from build123d import *

# Parameters (mm, degrees)
BOSS_EXTRUDE1_DEPTH     = 3
SKETCH2_R               = 0.875
CUT_EXTRUDE1_DEPTH      = 51
CUT_EXTRUDE1_DEPTH_BACK = 3
FILLET2_R               = 1.5
CHAMFER1_SIZE           = 1.5


with BuildPart() as part:
    # Sketch1 → Boss-Extrude1 (new body)
    with BuildSketch(Plane(origin=(0, 0, 0), x_dir=(1, 0, 0), z_dir=(0, 1, 0))):
        Polygon((-25, -21), (-20, -21), (-20, 11), (20, 11), (20, -21), (25, -21), (25, 14), (-25, 14), align=None)
    extrude(amount=BOSS_EXTRUDE1_DEPTH)

    # Sketch2 → Cut-Extrude1 (cut, two sides)
    with BuildSketch(Plane.ZY.offset(-25)) as cut_extrude1_sk:
        with Locations((18, 1.5)):
            Circle(SKETCH2_R)
        with Locations((13, 1.5)):
            Circle(SKETCH2_R)
        with Locations((8, 1.5)):
            Circle(SKETCH2_R)
        with Locations((3, 1.5)):
            Circle(SKETCH2_R)
        with Locations((-2, 1.5)):
            Circle(SKETCH2_R)
        with Locations((-7, 1.5)):
            Circle(SKETCH2_R)
    extrude(amount=CUT_EXTRUDE1_DEPTH, mode=Mode.SUBTRACT)
    extrude(cut_extrude1_sk.sketch, amount=-CUT_EXTRUDE1_DEPTH_BACK, mode=Mode.SUBTRACT)

    # Fillet2
    fillet2_edges = [part.edges().sort_by_distance(p)[0] for p in [
        (25, 1.5, 21),
        (-25, 1.5, 21),
        (-25, 1.5, -14),
        (25, 1.5, -14),
    ]]
    fillet(fillet2_edges, radius=FILLET2_R)

    # Chamfer1
    chamfer1_edges = [part.edges().sort_by_distance(p)[0] for p in [
        (20, 1.5, -11),
        (-20, 1.5, -11),
    ]]
    chamfer(chamfer1_edges, length=CHAMFER1_SIZE)


solid = part.part
Verification items for the finished model (mm, model axes). A direction names the side the tool comes from. Give positions to 0.01 mm unless a question says otherwise; leave off trailing zeros. Loops run counter-clockwise (first coordinate to the right, second up) from the corner with the lowest first, then second, coordinate; pieces in that order, holes last.
1) Thickness scan on line 1 along X through (y, z) = (0.7, 5); line 2 along Y through (x, z) = (22, 3) (3 decimals); line 3 along Z through (x, y) = (12, 1.8). Record the ranges inside material, lowest first.
2) Sectioned sample at B-B, the plane z = 8. Enter the section's corners in (x, y) (3 decimals).
3) Sectioned sample at C-C, the plane y = 1.5. Count the separate pieces of the cut face and the enclosed holes in it, then the cut area to 3 significant figures.
4) Depth check by flat-ended pin: pin 1 Ø1.5 at (x, y) = (-4, 2) entering from +Z. Enter the tip coordinate at first touch or a pass-through.
5) Set-up check for faces 1 (the flat face through (-6, 0, -12)), 2 (the flat face through (-20, 1, 6)): record each of +Z, -Z, +X, -X, +Y, -Y from which the full face is reachable in a straight line by a thin tool's end or side.
6) Sectioned sample at A-A, the plane z = 14.5. Enter the section's corners in (x, y), then the cut area to 3 significant figures.
7) Draft check along X on faces 3 (the flat face through (20, 1, 6)), 4 (the cylindrical face through (24.55, 1.52, 20.57)), 5 (the cylindrical face through (-22.465, 0.646, 2.81)). Enter one of: pulls with the +X half, pulls with the -X half, needs draft (parallel to the pull), parting line crosses it, or undercut.
8) Sectioned sample at D-D, the plane z = -10.5. Enter the section's corners in (x, y), then the cut area to 3 significant figures.
Answers:
1. line 1: x = -25 to -20, 20 to 25
1. line 2: y = 0 to 0.625, 2.375 to 3
1. line 3: z = -14 to -11
2. outline: (-25, 0) - (-20, 0) - (-20, 0.625) - (-25, 0.625) - close; (-25, 2.375) - (-20, 2.375) - (-20, 3) - (-25, 3) - close; (20, 0) - (25, 0) - (25, 0.625) - (20, 0.625) - close; (20, 2.375) - (25, 2.375) - (25, 3) - (20, 3) - close
3. separate pieces: 13
3. enclosed holes: 0
3. area: 365 mm2
4. pin 1: stops at z = -11
5. face 1: +Z, -Z, +X, -X, -Y
5. face 2: +Z, +Y, -Y
6. outline: (-25, 0) - (-20, 0) - (-20, 3) - (-25, 3) - close; (20, 0) - (25, 0) - (25, 3) - (20, 3) - close
6. area: 30.0 mm2
7. face 3: undercut
7. face 4: pulls with the +X half
7. face 5: needs draft
8. outline: (-25, 0) - (-19, 0) - (-19, 3) - (-25, 3) - close; (19, 0) - (25, 0) - (25, 3) - (19, 3) - close
8. area: 36.0 mm2
